Model file for the job. Use its own axes, mm. A direction names the side the tool comes from. Round coordinates to 2 decimals unless told otherwise and drop trailing zeros. Order: outer loops, then holes, each group sorted by start corner. A loop starts at its lowest first (then second) coordinate and runs counter-clockwise, first axis right, second up. Notation, with made-up numbers: (51.25, -2.5) -> (92.25, -2.5) arc R18 cw to (92.25, 32.5) -> close; hole circle Ø7 at (50.25, 47.25). An arc over 180 degrees is marked (long way). Use CSV: the item, a comma, the result in double quotes.
```python
from build123d import *

# Parameters (mm, degrees)
MODEL_W             = 20
MODEL_H             = 3
BOSS_EXTRUDE1_DEPTH = 3


with BuildPart() as part:
    # Model → Boss-Extrude1 (new body)
    with BuildSketch(Plane.XY):
        Polygon((149.457182746, 55.697979038), (120.785258916, 105.359207863), (63.441411255, 105.359207863), (34.769487424, 55.697979038), (63.441411255, 6.036750213), (120.785258916, 6.036750213), align=None)
        with Locations((92.113335085, 102.359207863)):
            Rectangle(MODEL_W, MODEL_H, mode=Mode.SUBTRACT)
        with Locations((92.113335085, 9.036750213)):
            Rectangle(MODEL_W, MODEL_H, mode=Mode.SUBTRACT)
        Polygon((126.215627262, 24.442424093), (128.813703474, 22.942424093), (138.813703474, 40.262932169), (136.215627262, 41.762932169), align=None, mode=Mode.SUBTRACT)
        Polygon((128.839141228, 88.429056492), (126.241065016, 86.929056492), (136.241065016, 69.608548416), (138.839141228, 71.108548416), align=None, mode=Mode.SUBTRACT)
        Polygon((55.387528943, 22.927737599), (57.985605154, 24.427737599), (47.985605154, 41.748245675), (45.387528943, 40.248245675), align=None, mode=Mode.SUBTRACT)
        Polygon((45.387528943, 71.108548416), (47.985605154, 69.608548416), (57.985605154, 86.929056492), (55.387528943, 88.429056492), align=None, mode=Mode.SUBTRACT)
    extrude(amount=BOSS_EXTRUDE1_DEPTH)


solid = part.part
```
Q1. Which spindle directions (+Z, -Z, +X, -X, +Y, -Y) get a long thin tool onto all of the face, cutting with end or side? Do faces 1 (the flat face through (127.56, 87.69, 1.48)), 2 (the flat face through (93, 105.359, 1)). Say none if no direction does.
From the geometry:
face 1,"+Z, -Z"
face 2,"+Z, -Z, +X, -X, +Y"
Q2. Probe line 1 along Y through (x, z) = (89.5, 1.4); line 2 along Y through (x, z) = (133, 1.9); line 3 along X through (y, z) = (86, 1.25). List the from-to ranges inside material, lowest first.
From the geometry:
line 1,"y = 6.04 to 7.54, 10.54 to 100.86, 103.86 to 105.36"
line 2,"y = 27.19 to 30.19, 36.19 to 75.22, 81.22 to 84.2"
line 3,"x = 52.26 to 53.99, 57.45 to 126.78, 130.24 to 131.96"
Q3. Cut at B-B (y = 81.5). Give the cut face in (x, z).
From the geometry:
outline,"(49.67, 0) -> (51.39, 0) -> (51.39, 3) -> (49.67, 3) -> close; (54.85, 0) -> (129.38, 0) -> (129.38, 3) -> (54.85, 3) -> close; (132.84, 0) -> (134.56, 0) -> (134.56, 3) -> (132.84, 3) -> close"
Q4. Cut at D-D (y = 53). Give the cut face in (x, z).
From the geometry:
outline,"(36.33, 0) -> (147.9, 0) -> (147.9, 3) -> (36.33, 3) -> close"
Q5. Cut at A-A (x = 95). Give the cut face in (y, z).
From the geometry:
outline,"(6.04, 0) -> (7.54, 0) -> (7.54, 3) -> (6.04, 3) -> close; (10.54, 0) -> (100.86, 0) -> (100.86, 3) -> (10.54, 3) -> close; (103.86, 0) -> (105.36, 0) -> (105.36, 3) -> (103.86, 3) -> close"
Q6. Pin check, flat tips, straight feed: pin 1 (1.5 mm diameter, centred on y = 101.5, z = 1, fed in from -X); pin 2 (1.5 mm diameter, centred on y = 9.5, z = 1, fed in from -X); pin 3 (1.5 mm diameter, centred on y = 9.5, z = 1, fed in from +X). Stop position of each tip, or through.
From the geometry:
pin 1,"stops at x = 60.78"
pin 2,"stops at x = 61.01"
pin 3,"stops at x = 123.22"
Q7. Cut at C-C (z = 1.3). State how many separate pieces and enclosed holes the cut face has, plus the area to 3 significant figures.
From the geometry:
separate pieces,"1"
enclosed holes,"6"
area,"8,180 mm²"
Q8. Mould opens along X. For faces 3 (the flat face through (91, 56, 0)), 4 (the flat face through (56.7, 87.67, 1.48)), 5 (the flat face through (135.322, 80.181, 1.479)) say: +X half, -X half, draft (parallel to the pull), parting line (faces both ways), or undercut.
From the geometry:
face 3,"draft"
face 4,"undercut"
face 5,"+X half"
